Autodesk Inventor part; units mm, degrees
ref_plane "YZ Plane" through (0, 0, 0) normal (1, 0, 0) x (0, 1, 0)
ref_plane "XZ Plane" through (0, 0, 0) normal (0, 1, 0) x (-1, 0, 0)
ref_plane "XY Plane" through (0, 0, 0) normal (0, 0, 1) x (1, 0, 0)
sketch "スケッチ1" plane through (0, 0, 0) normal (0, 0, 1) x (1, 0, 0)
  line L0 (2.8284, 0) -> (0, -2.8284)
  line L1 (0, -2.8284) -> (-2.8284, 0)
  line L2 (-2.8284, 0) -> (0, 2.8284)
  line L3 (0, 2.8284) -> (2.8284, 0)
  line L4 (-12.1149, 7.5) -> (-10, -7.5)
  line L5 (10, -7.5) -> (-10, -7.5)
  line L6 (10, -7.5) -> (12.1149, 7.5)
  line L7 (12.1149, 7.5) -> (-12.1149, 7.5)
  point P0 (0, 0)
  point P1 (0, 7.5)
  point P2 (11.0574, 0)
  dimension "d10" = 24.2298
  dimension "d11" = 20
  dimension "d12" = 15
  dimension "d13" = 4
extrude "押し出し1" add sketch "スケッチ1" against normal blind 2
sketch "スケッチ2" plane through (0, 0, 0) normal (0, 0, 1) x (1, 0, 0)
  line L0 (10, -7.5) -> (13.8567, -12.0963)
  line L1 (13.8567, -12.0963) -> (11.0574, 0)
  line L2 (-12.1149, 7.5) -> (12.1149, 7.5)
  line L3 (12.1149, 7.5) -> (10, -7.5)
  line L4 (10, -7.5) -> (-10, -7.5)
  line L5 (-10, -7.5) -> (-12.1149, 7.5)
  line L6 (0, -2.8284) -> (2.8284, 0)
  line L7 (2.8284, 0) -> (0, 2.8284)
  line L8 (0, 2.8284) -> (-2.8284, 0)
  line L9 (-2.8284, 0) -> (0, -2.8284)
  dimension "d7" = 6
  dimension "d14" = 130
extrude "押し出し2" add sketch "スケッチ2" against normal up to surface (2 mm away) contours L3 L1 L0
mirror "ミラー1" about plane through (0, 0, 0) normal (1, 0, 0) of "押し出し2"
properties part number "om_BackHolder_V2"
Work out the finished part from the listing and answer in its coordinate system (mm). A direction names the side the tool comes from. Round coordinates to 2 decimals unless told otherwise and drop trailing zeros. Write each loop counter-clockwise with the first axis right and the second up, starting at its lowest first coordinate (ties: lowest second). Pieces come first, ordered by that corner, then holes.
1) A cutting plane is placed at C-C (z = -0.95). Give the vertices of the cut face in (x, y).
2) A cutting plane is placed at A-A (y = -0.5). Give the vertices of the cut face in (x, z), plus the area to 3 significant figures.
3) A tool of negligible diameter and unlimited length cuts with its end or side. For faces 4 (the flat face through (-12.437, -5.963, -0.986)), 5 (the flat face through (3, 0, -2)), 6 (the flat face through (11.901, -9.766, -0.986)), 7 (the flat face through (1.434, -1.394, -0.986)), 8 (the flat face through (11.58, 3.7, -0.99)), from which of +Z, -Z, +X, -X, +Y, -Y can it reach the whole face along a straight path? Write none if from no direction.
4) The mould has two halves that part along Y. Classify faces 1 (the flat face through (3, 0, 0)), 2 (the flat face through (-11.955, -9.83, -0.986)), 3 (the flat face through (12.477, -6.133, -0.986)): pulls with the +Y half, pulls with the -Y half, needs draft (parallel to the pull), parting line crosses it, or undercut.
5) A cutting plane is placed at B-B (x = 1). Give the vertices of the cut face in (y, z).
6) A cutting plane is placed at D-D (x = 7.5). Give the vertices of the cut face in (y, z).
7) Straight lines are drawn through the part: line 1 (Y direction, x = 5, z = -1.2); line 2 (X direction, y = -9.75, z = -0.9); line 3 (X direction, y = -8, z = -1.8). For each, find the intervals that lie inside material, in ascending order.
8) Given pin 1 Ø1 at (x, z) = (-2.5, -1) entering from -Y; pin 2 Ø1 at (y, z) = (3, -1.5) entering from -X, each flat-ended and moving along its own axis, determine where each tip first touches the part or whether it passes through.
Completed:
1. outline: (-13.86, -12.1) - (-10, -7.5) - (10, -7.5) - (13.86, -12.1) - (11.06, 0) - (12.11, 7.5) - (-12.11, 7.5) - (-11.06, 0) - close; hole (-2.83, 0) - (0, -2.83) - (2.83, 0) - (0, 2.83) - close
2. outline: (-11.17, -2) - (-2.33, -2) - (-2.33, 0) - (-11.17, 0) - close; (2.33, -2) - (11.17, -2) - (11.17, 0) - (2.33, 0) - close
2. area: 35.4 mm2
3. face 4: +Z, -Z, -X
3. face 5: -Z, +X, -X, +Y, -Y
3. face 6: +Z, -Z, -Y
3. face 7: +Z, -Z
3. face 8: +Z, -Z, +X
4. face 1: needs draft
4. face 2: pulls with the -Y half
4. face 3: undercut
5. outline: (-7.5, -2) - (-1.83, -2) - (-1.83, 0) - (-7.5, 0) - close; (1.83, -2) - (7.5, -2) - (7.5, 0) - (1.83, 0) - close
6. outline: (-7.5, -2) - (7.5, -2) - (7.5, 0) - (-7.5, 0) - close
7. line 1: y = -7.5 to 7.5
7. line 2: x = -13.31 to -11.89, 11.89 to 13.31
7. line 3: x = -12.91 to -10.42, 10.42 to 12.91
8. pin 1: stops at y = -7.5
8. pin 2: stops at x = -11.55
